Input: dimensioned drawing with shaded views. Units: mm. Origin: part minimum x, y, z. A direction names the side the tool comes from. Give positions to 0.01 mm unless a question says otherwise; leave off trailing zeros. Write each loop counter-clockwise with the first axis right and the second up, starting at its lowest first coordinate (ties: lowest second). Pieces come first, ordered by that corner, then holes. Notation, with made-up numbers: M 38,86 L 52,86 A26 cw 52,105 Z; hole C 73.25,20.25 d3. An arc over 180 degrees is marked long. Answer as a JSON object with one key per item and string values.
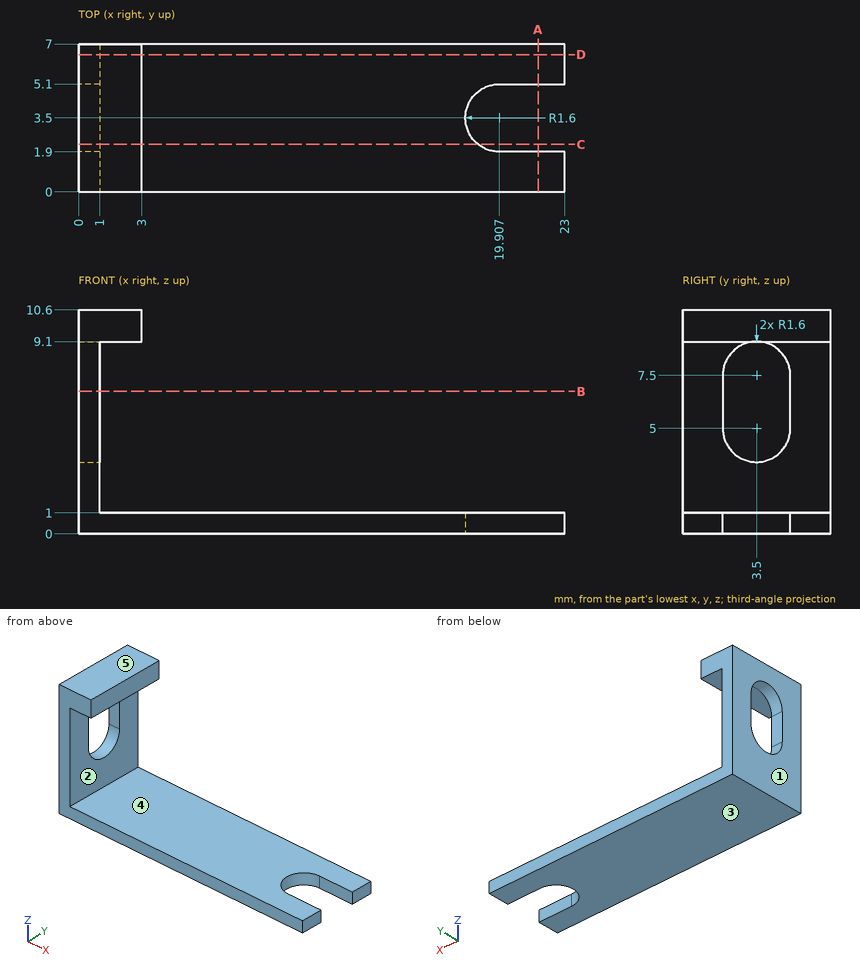
1) Cut plane C-C on y = 2.25. Return loops of the section in (x, z), and give its area (3 significant figures).
Geometry check:
{"outline": "M 0,0 L 18.91,0 L 18.91,1 L 1,1 L 1,4 L 0,4 Z; M 0,8.5 L 1,8.5 L 1,9.1 L 3,9.1 L 3,10.6 L 0,10.6 Z", "area": "27.0 mm2"}
2) Contact query for a flat-ended pin moving along its axis: P1, Ø3.5, axis at y = 3.5, z = 5, coming from the +X side. Output: stop coordinate, or through.
Geometry check:
{"P1": "stops at x = 1"}
3) Pull-direction query (Z, two-part tool) for the marked faces 1, 2 and 3; classes: pulls with the +Z half, pulls with the -Z half, needs draft (parallel to the pull), parting line crosses it, or undercut.
Geometry check:
{"face 1": "needs draft", "face 2": "undercut", "face 3": "pulls with the -Z half"}
4) Cut plane D-D on y = 6.5. Return loops of the section in (x, z), and give its area (3 significant figures).
Geometry check:
{"outline": "M 0,0 L 23,0 L 23,1 L 1,1 L 1,9.1 L 3,9.1 L 3,10.6 L 0,10.6 Z", "area": "35.6 mm2"}
5) Cut plane B-B on z = 6.75. Return loops of the section in (x, y), and give its area (3 significant figures).
Geometry check:
{"outline": "M 0,0 L 1,0 L 1,1.9 L 0,1.9 Z; M 0,5.1 L 1,5.1 L 1,7 L 0,7 Z", "area": "3.80 mm2"}
6) Set-up query: the marked faces 4 and 5. Return all of +Z, -Z, +X, -X, +Y, -Y with unobstructed straight access to the full face (end or side cutting, diameter ignored); none if empty.
Geometry check:
{"face 4": "+X, +Y, -Y", "face 5": "+Z, +X, -X, +Y, -Y"}
7) Line query: line 1 (X direction, y = 2, z = 2); line 2 (X direction, y = 3.5, z = 9.75). Output: solid intervals per line, ascending. Write a range as from..to.
Geometry check:
{"line 1": "x = 0..1", "line 2": "x = 0..3"}
8) Cut plane A-A on x = 21.75. Return loops of the section in (y, z), and give its area (3 significant figures).
Geometry check:
{"outline": "M 0,0 L 1.9,0 L 1.9,1 L 0,1 Z; M 5.1,0 L 7,0 L 7,1 L 5.1,1 Z", "area": "3.80 mm2"}
